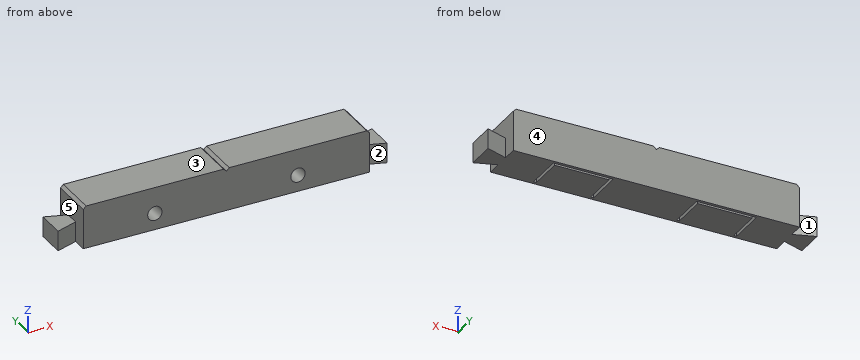
```python
from build123d import *

# Parameters (mm, degrees)
SKETCH1_W              = 100
SKETCH1_H              = 15
BODY_DEPTH             = 15
CLICK_DEPTH            = 7
CLICK_CHAMFER_SIZE     = 1
SKETCH3_R              = 2.5
LED_HOLE_DEPTH         = 8
SKETCH4_W              = 2
SKETCH4_H              = 15
FIELDMARK_DEPTH        = 2
FIELDMARK_CHAMFER_SIZE = 2
LIGHT_START            = -1
SKETCH6_W              = 1
SKETCH6_H              = 15
LIGHT_GUIDE_DEPTH      = 13
SKETCH7_W              = 19
SKETCH7_H              = 1
CUT_EXTRUDE1_DEPTH     = 13.25


with BuildPart() as part:
    # Sketch1 → Body (new body)
    with BuildSketch(Plane.XY):
        Rectangle(SKETCH1_W, SKETCH1_H)
    extrude(amount=BODY_DEPTH)

    # Sketch2 → Click (add)
    with BuildSketch(Plane.XY):
        Polygon((-50, 0), (-50, 2.45), (-57.45, 4.95), (-57.45, 0), (-57.45, -4.95), (-50, -2.45), align=None)
        Polygon((57.45, 0), (57.45, -4.95), (50, -2.45), (50, 0), (50, 2.45), (57.45, 4.95), align=None)
    extrude(amount=CLICK_DEPTH)

    # Click Chamfer
    click_chamfer_edges = [part.edges().sort_by_distance(p)[0] for p in [
        (-50, 0, 15),
        (50, 0, 15),
    ]]
    chamfer(click_chamfer_edges, length=CLICK_CHAMFER_SIZE)

    # Sketch3 → LED Hole (cut)
    with BuildSketch(Plane.XZ.offset(7.5)):
        with Locations(Location((-25, 5.75, 0), (0, 0, 270))):
            Circle(SKETCH3_R)
        with Locations(Location((25, 5.75, 0), (0, 0, 270))):
            Circle(SKETCH3_R)
    extrude(amount=-LED_HOLE_DEPTH, mode=Mode.SUBTRACT)

    # Sketch4 → FieldMark (cut)
    with BuildSketch(Plane.XY.offset(15)):
        Rectangle(SKETCH4_W, SKETCH4_H)
    extrude(amount=-FIELDMARK_DEPTH, mode=Mode.SUBTRACT)

    # FieldMark Chamfer
    # the kernel refuses this chamfer: 2 mm, written as the material it adds along each edge
    with BuildSketch(Plane(origin=(1, -7.5, 13), x_dir=(0.02749587661058638, 0, 0.9996219169112968), z_dir=(0, 1, 0))) as fieldmark_chamfer_piece_1_section:
        Polygon((FIELDMARK_CHAMFER_SIZE * 0.999621916911, -FIELDMARK_CHAMFER_SIZE * 0.0274958766106), (-FIELDMARK_CHAMFER_SIZE * 0.0274958766106, -FIELDMARK_CHAMFER_SIZE * 0.999621916911), (0, 0), align=None)
    fieldmark_chamfer_piece_1 = extrude(amount=15, mode=Mode.PRIVATE)
    fieldmark_chamfer_piece_1 = split(fieldmark_chamfer_piece_1, bisect_by=Plane(origin=(0.339191691, 0, 15), z_dir=(0, 0, -1)), keep=Keep.TOP, mode=Mode.PRIVATE)
    add(fieldmark_chamfer_piece_1)
    with BuildSketch(Plane(origin=(-1, 7.5, 13), x_dir=(0.9996219169112968, 0, -0.027495876610586487), z_dir=(0, -1, 0))) as fieldmark_chamfer_piece_2_section:
        Polygon((FIELDMARK_CHAMFER_SIZE * 0.999621916911, FIELDMARK_CHAMFER_SIZE * 0.0274958766106), (-FIELDMARK_CHAMFER_SIZE * 0.0274958766106, FIELDMARK_CHAMFER_SIZE * 0.999621916911), (0, 0), align=None)
    fieldmark_chamfer_piece_2 = extrude(amount=15, mode=Mode.PRIVATE)
    fieldmark_chamfer_piece_2 = split(fieldmark_chamfer_piece_2, bisect_by=Plane(origin=(-0.339191691, 0, 15), z_dir=(0, 0, -1)), keep=Keep.TOP, mode=Mode.PRIVATE)
    add(fieldmark_chamfer_piece_2)

    # Sketch6 → Light Guide (cut)
    with BuildSketch(Plane.XZ.offset(7.5).offset(LIGHT_START)):
        with Locations((35, 5.75)):
            Rectangle(SKETCH6_W, SKETCH6_H)
        with Locations((15, 5.75)):
            Rectangle(SKETCH6_W, SKETCH6_H)
        with Locations((-15, 5.75)):
            Rectangle(SKETCH6_W, SKETCH6_H)
        with Locations((-35, 5.75)):
            Rectangle(SKETCH6_W, SKETCH6_H)
    extrude(amount=-LIGHT_GUIDE_DEPTH, mode=Mode.SUBTRACT)

    # Sketch7 → Cut-Extrude1 (cut)
    with BuildSketch(Plane(origin=(0, 0, 0), x_dir=(-1, 0, 0), z_dir=(0, 0, -1))):
        with Locations((25, 6)):
            Rectangle(SKETCH7_W, SKETCH7_H)
        with Locations((-25, 6)):
            Rectangle(SKETCH7_W, SKETCH7_H)
    extrude(amount=-CUT_EXTRUDE1_DEPTH, mode=Mode.SUBTRACT)


solid = part.part
```
Geometry check sheet. Reference: the model listing, model coordinates, mm. Face numbers are marked on the shaded views. A direction names the side the tool comes from. Round coordinates to 2 decimals unless told otherwise and drop trailing zeros. Order: outer loops, then holes, each group sorted by start corner. A loop starts at its lowest first (then second) coordinate and runs counter-clockwise, first axis right, second up. Notation, with made-up numbers: (-0.5, 45) - (50.5, 45) arc R23 cw to (50.5, 82) - close; hole circle Ø9 at (50, -16.75). An arc over 180 degrees is marked (long way). Use a Markdown table: item, result. Add a question column.
(1) Depth check by flat-ended pin: pin 1 (6 mm diameter, centred on x = -55.5, y = -0.5, fed in from +Z); pin 2 (1.5 mm diameter, centred on x = -26, z = 5.5, fed in from -Y). Enter the tip coordinate at first touch or a pass-through.
(2) Sectioned sample at B-B, the plane x = 30. Enter the section's corners in (y, z), and give its area (3 significant figures).
(3) Tool access check on the marked faces 1, 2 and 3. Record the directions out of +Z, -Z, +X, -X, +Y, -Y that give a thin tool (end or side, any length) a straight path to the whole face; none if there is none.
(4) Sectioned sample at C-C, the plane z = 1.75. Enter the section's corners in (x, y).
(5) Release check for a two-part mould opening along X. For the marked faces 4 and 5 record: pulls with the +X half, pulls with the -X half, needs draft (parallel to the pull), parting line crosses it, or undercut.
(6) Material ranges on line 1 along X through (y, z) = (-1, 1.75); line 2 along X through (y, z) = (5.25, 1.5); line 3 along X through (y, z) = (5.75, 10), recorded low to high. Write a range as [from, to].
(7) Sectioned sample at D-D, the plane y = -4. Count the separate pieces of the cut face and the enclosed holes in it, and give its area (3 significant figures).
(8) Sectioned sample at A-A, the plane z = 12.25. Enter the section's corners in (x, y), and give its area (3 significant figures).
Answers below:
| question | item | result |
|---|---|---|
| 1 | pin 1 | z = 7 |
| 1 | pin 2 | y = 0.5 |
| 2 | outline | (-7.5, 0) - (5.5, 0) - (5.5, 13.25) - (6.5, 13.25) - (6.5, 0) - (7.5, 0) - (7.5, 15) - (-7.5, 15) - close |
| 2 | area | 212 mm² |
| 3 | face 1 | +Z, -Z, +Y |
| 3 | face 2 | +Z, -Z, -Y |
| 3 | face 3 | +Z, +X, -X, +Y, -Y |
| 4 | outline | (-57.45, -4.95) - (-50, -2.45) - (-50, -7.5) - (50, -7.5) - (50, -2.45) - (57.45, -4.95) - (57.45, 4.95) - (50, 2.45) - (50, 7.5) - (-50, 7.5) - (-50, 2.45) - (-57.45, 4.95) - close; hole (-35.5, -6.5) - (-34.5, -6.5) - (-34.5, 5.5) - (-15.5, 5.5) - (-15.5, -6.5) - (-14.5, -6.5) - (-14.5, 6.5) - (-35.5, 6.5) - close; hole (14.5, -6.5) - (15.5, -6.5) - (15.5, 5.5) - (34.5, 5.5) - (34.5, -6.5) - (35.5, -6.5) - (35.5, 6.5) - (14.5, 6.5) - close |
| 5 | face 4 | needs draft |
| 5 | face 5 | undercut |
| 6 | line 1 | [-57.45, -35.5], [-34.5, -15.5], [-14.5, 14.5], [15.5, 34.5], [35.5, 57.45] |
| 6 | line 2 | [-50, -35.5], [-34.5, -15.5], [-14.5, 14.5], [15.5, 34.5], [35.5, 50] |
| 6 | line 3 | [-50, -35.5], [-14.5, 14.5], [35.5, 50] |
| 7 | separate pieces | 3 |
| 7 | enclosed holes | 2 |
| 7 | area | 1,450 mm² |
| 8 | outline | (-50, -7.5) - (50, -7.5) - (50, 7.5) - (-50, 7.5) - close; hole (-35.5, -6.5) - (-34.5, -6.5) - (-34.5, 5.5) - (-15.5, 5.5) - (-15.5, -6.5) - (-14.5, -6.5) - (-14.5, 6.5) - (-35.5, 6.5) - close; hole (14.5, -6.5) - (15.5, -6.5) - (15.5, 5.5) - (34.5, 5.5) - (34.5, -6.5) - (35.5, -6.5) - (35.5, 6.5) - (14.5, 6.5) - close |
| 8 | area | 1,410 mm² |
